Can you work these out from the model? Positions are in its coordinate system, mm. Face numbers are marked on the shaded views. A direction names the side the tool comes from. Round coordinates to 2 decimals unless told otherwise and drop trailing zeros. Loops run counter-clockwise (first coordinate to the right, second up) from the corner with the lowest first, then second, coordinate; pieces in that order, holes last. Notation, with made-up numbers: (-14, -36) -> (45, -36) arc R24 cw to (45, -19) -> close; hole circle Ø9 at (29.5, 34). An arc over 180 degrees is marked (long way). Use a Markdown table: item, result.
Autodesk Inventor part; units mm, degrees
ref_plane "YZ Plane" through (0, 0, 0) normal (1, 0, 0) x (0, 1, 0)
ref_plane "XZ Plane" through (0, 0, 0) normal (0, 1, 0) x (-1, 0, 0)
ref_plane "XY Plane" through (0, 0, 0) normal (0, 0, 1) x (1, 0, 0)
sketch "Esquisse1" plane through (0, 0, 0) normal (0, 1, 0) x (-1, 0, 0)
  line L0 (-20, 5.3) -> (20, 5.3)
  line L1 (20, 5.3) -> (20, -5.3)
  line L2 (20, -5.3) -> (-20, -5.3)
  line L3 (-20, -5.3) -> (-20, 5.3)
  point P0 (0, 0)
  dimension "d0" = 40
  dimension "d1" = 10.6
  dimension "d2" = 20
  dimension "d3" = 5.3
extrude "Extrusion1" add sketch "Esquisse1" along normal blind 11.6
sketch "Esquisse2" plane through (20, 0, 5.3) normal (1, 0, 0) x (0, 0, -1)
  line L0 (2.55, 9.05) -> (8.05, 9.05)
  line L1 (8.05, 9.05) -> (8.05, 2.55)
  line L2 (8.05, 2.55) -> (2.55, 2.55)
  line L3 (2.55, 2.55) -> (2.55, 9.05)
  point P0 (0, 11.6)
  point P1 (5.3, 0)
  dimension "d6" = 5.5
  dimension "d8" = 2.75
  dimension "d9" = 6.5
  dimension "d10" = 2.55
extrude "Extrusion2" cut sketch "Esquisse2" against normal blind 8
sketch "Esquisse3" plane through (-20, 0, -5.3) normal (-1, 0, 0) x (0, 0, 1)
  line L0 (2.55, 9.05) -> (8.05, 9.05)
  line L1 (8.05, 9.05) -> (8.05, 2.55)
  line L2 (8.05, 2.55) -> (2.55, 2.55)
  line L3 (2.55, 2.55) -> (2.55, 9.05)
  point P0 (0, 11.6)
  point P1 (5.3, 0)
  dimension "d13" = 5.5
  dimension "d14" = 6.5
  dimension "d15" = 2.75
  dimension "d16" = 2.55
extrude "Extrusion3" cut sketch "Esquisse3" against normal blind 8
sketch "Esquisse4" plane through (-12, 0, -5.3) normal (-1, 0, 0) x (0, 0, 1)
  line L0 (2.55, 9.05) -> (8.05, 9.05)
  line L1 (2.55, 2.55) -> (2.55, 9.05)
  circle A0 centre (5.3, 5.8) radius 1.25
  point P0 (5.3, 0)
  dimension "d19" = 2.5
  dimension "d20" = 3.25
  dimension "d21" = 2.75
extrude "Extrusion4" cut sketch "Esquisse4" against normal through all
sketch "Esquisse5" plane through (0, 11.6, 0) normal (0, 1, 0) x (1, 0, 0)
  circle A0 centre (0, 0) radius 1.25
  dimension "d24" = 2.5
extrude "Extrusion5" cut sketch "Esquisse5" against normal through all
equation "\"d20\" = 0.5 * d14"
properties part number "Truc Lumiere"
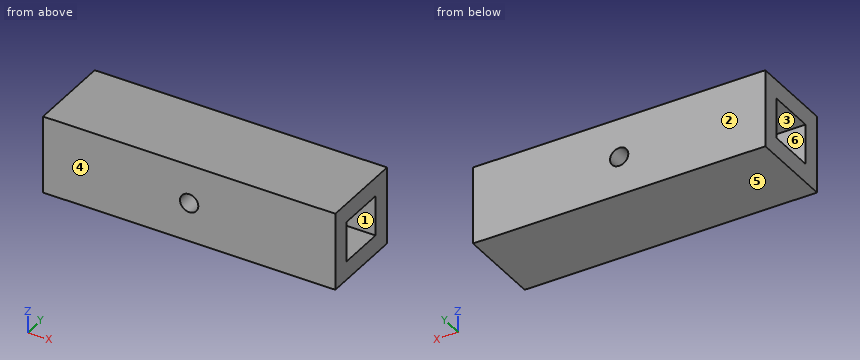
1. Will these pins go through, and if not, where does the flat tip stop? pin 1 Ø6 at (x, z) = (15.5, 0) entering from -Y; pin 2 Ø2 at (x, z) = (0, 0) entering from +Y; pin 3 Ø3 at (y, z) = (7, -0.5) entering from -X; pin 4 Ø4 at (y, z) = (5.8, 0) entering from +X.
Answer sheet:
| item | result |
|---|---|
| pin 1 | stops at y = 0 |
| pin 2 | passes through |
| pin 3 | stops at x = -12 |
| pin 4 | stops at x = 12 |
2. I want a section at D-D (z = -2.25). Please give me the cut outline in (x, y).
Answer sheet:
| item | result |
|---|---|
| outline | (-20, 0) -> (20, 0) -> (20, 2.55) -> (12, 2.55) -> (12, 9.05) -> (20, 9.05) -> (20, 11.6) -> (-20, 11.6) -> (-20, 9.05) -> (-12, 9.05) -> (-12, 2.55) -> (-20, 2.55) -> close |
3. I want a section at A-A (z = 0). Please give me the cut outline in (x, y).
Answer sheet:
| item | result |
|---|---|
| outline | (-20, 0) -> (-1.25, 0) -> (-1.25, 4.55) -> (-12, 4.55) -> (-12, 2.55) -> (-20, 2.55) -> close; (-20, 9.05) -> (-12, 9.05) -> (-12, 7.05) -> (-1.25, 7.05) -> (-1.25, 11.6) -> (-20, 11.6) -> close; (1.25, 0) -> (20, 0) -> (20, 2.55) -> (12, 2.55) -> (12, 4.55) -> (1.25, 4.55) -> close; (1.25, 7.05) -> (12, 7.05) -> (12, 9.05) -> (20, 9.05) -> (20, 11.6) -> (1.25, 11.6) -> close |
4. I need wall thicknesses on line 1 (Z direction, x = -12.5, y = 3); line 2 (Z direction, x = 0, y = 3.85); line 3 (Y direction, x = 4, z = 0). Which ranges of each line are inside material? Lowest first, please.
Answer sheet:
| item | result |
|---|---|
| line 1 | z = -5.3 to -2.75, 2.75 to 5.3 |
| line 2 | z = -5.3 to -1.25, 1.25 to 5.3 |
| line 3 | y = 0 to 4.55, 7.05 to 11.6 |
5. I want a section at B-B (x = -15.5). Please give me the cut outline in (y, z), plus the area to 3 significant figures.
Answer sheet:
| item | result |
|---|---|
| outline | (0, -5.3) -> (11.6, -5.3) -> (11.6, 5.3) -> (0, 5.3) -> close; hole (2.55, -2.75) -> (9.05, -2.75) -> (9.05, 2.75) -> (2.55, 2.75) -> close |
| area | 87.2 mm² |
6. If we mould it in two halves opening along Y, with no side actions, what happens to the marked faces 3, 4, 5 and 6? For each: +Y half, -Y half, draft (parallel to the pull), parting line (faces both ways), or undercut.
Answer sheet:
| item | result |
|---|---|
| face 3 | undercut |
| face 4 | -Y half |
| face 5 | draft |
| face 6 | undercut |
7. Which directions (+Z, -Z, +X, -X, +Y, -Y) give clear straight access to the entire face, cutting with the end or side of a thin tool? Please do the marked faces 1 and 2.
Answer sheet:
| item | result |
|---|---|
| face 1 | +X |
| face 2 | +Z, -Z, +X, -X, +Y |
8. I want a section at C-C (y = 4). Please give me the cut outline in (x, z), plus the area to 3 significant figures.
Answer sheet:
| item | result |
|---|---|
| outline | (-20, -5.3) -> (20, -5.3) -> (20, -2.75) -> (12, -2.75) -> (12, 2.75) -> (20, 2.75) -> (20, 5.3) -> (-20, 5.3) -> (-20, 2.75) -> (-12, 2.75) -> (-12, -2.75) -> (-20, -2.75) -> close; hole circle Ø2.5 at (0, 0) |
| area | 331 mm² |
